```python
from build123d import *

# Parameters (mm, degrees)
F1_DEPTH = 870
F2_T     = -7


with BuildPart() as f1:
    # F0 (on Top) → F1 (new body)
    with BuildSketch(Plane.XY):
        Polygon((13.739455, 85.505716), (-80.919849, -30.854141), (67.180395, -54.651574), align=None)
    extrude(amount=F1_DEPTH)

    # F2
    f2_openings = [f1.faces().sort_by_distance(p)[0] for p in [
        (0, 0, 870),
    ]]
    offset(amount=F2_T, openings=f2_openings)


solid = f1.part
```
Can you work these out from the model? Positions are in its coordinate system, mm. A direction names the side the tool comes from. Coordinates: 2 decimals unless noted, no trailing zeros. Loops run counter-clockwise (first coordinate to the right, second up) from the corner with the lowest first, then second, coordinate; pieces in that order, holes last. Notation, with made-up numbers: M 48,6.25 L 67,6.25 A30 ccw 67,37.25 Z; hole C 16.25,74 d1. An arc over 180 degrees is marked long. Put each result on its own line as item: value. Start each with the question number.
(1) Imagine slicing it at B-B on x = -15. List the corners of the cut face in (y, z) for me.
(2) Imagine slicing it at C-C on y = 46. List the corners of the cut face in (x, z) for me, and give its area (3 significant figures).
(3) Imagine slicing it at A-A on z = 354.5. List the corners of the cut face in (x, y) for me.
(4) Will these pins go through, and if not, where does the flat tip stop? pin 1 Ø2 at (y, z) = (54.5, 629) entering from +X; pin 2 Ø3 at (x, z) = (-3, 551.5) entering from +Y; pin 3 Ø2 at (x, z) = (32.5, 432.5) entering from -Y.
(5) We'd pull the mould along Y, two halves only. Please class faces 3 (the face through (-7.906, -42.586, 428.91)), 4 (the face through (-7, 1, 7)), 5 (the face through (40.834, 14.446, 428.91)): +Y half, -Y half, draft (parallel to the pull), parting line (faces both ways), or undercut.
(6) Which directions (+Z, -Z, +X, -X, +Y, -Y) give clear straight access to the entire face, cutting with the end or side of a thin tool? Please do faces 1 (the face through (-6.63, -35.7, 432.46)), 2 (the face through (-7, -36, 870)).
(7) I need wall thicknesses on probe 1 along Z at (x, y) = (17, 26); probe 2 along Y at (x, z) = (-28.5, 442.5); probe 3 along X at (y, z) = (48.5, 521.5). Which ranges of each line are inside material? Lowest first, please.
Worked answers:
1. outline: M -41.45,0 L 50.18,0 L 50.18,870 L 39.09,870 L 39.09,7 L -34.36,7 L -34.36,870 L -41.45,870 Z
2. outline: M -18.4,0 L 28.8,0 L 28.8,870 L 21.31,870 L 21.31,7 L -9.37,7 L -9.37,870 L -18.4,870 Z
2. area: 14,600 mm2
3. outline: M -80.92,-30.85 L 67.18,-54.65 L 13.74,85.51 Z; hole M -67.84,-25.87 L 56.32,-45.82 L 11.52,71.68 Z
4. pin 1: stops at x = 25.94
4. pin 2: stops at y = 66.77
4. pin 3: stops at y = -49.24
5. face 3: -Y half
5. face 4: undercut
5. face 5: +Y half
6. face 1: +Z
6. face 2: +Z, +X, -X, +Y, -Y
7. probe 1: z = 0 to 7
7. probe 2: y = -39.28 to -32.19, 22.49 to 33.58
7. probe 3: x = -16.36 to -7.34, 20.36 to 27.85
